Design review of the part shown in the three views and the two pictorial views. Dimensions are in mm from the part's minimum x, y and z. Round coordinates to 2 decimals unless told otherwise and drop trailing zeros. Order: outer loops, then holes, each group sorted by start corner. A loop starts at its lowest first (then second) coordinate and runs counter-clockwise, first axis right, second up.
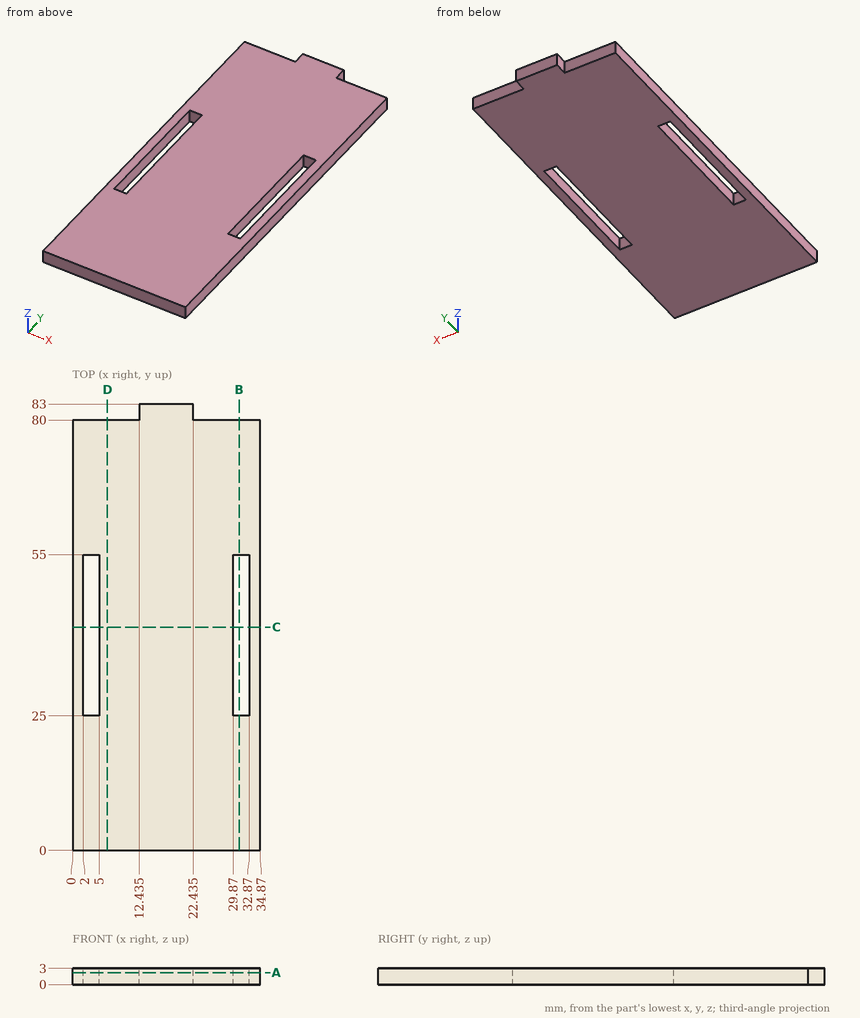
(1) Add section B-B on x = 31. Give the boundary of the cut face in (y, z).
(2) Add section A-A on z = 2.2. Give the boundary of the cut face in (x, y) (3 decimals), plus the area to 3 significant figures.
(3) Clearance check with flat-ended pins moving along their axes: P1, Ø0.9, axis at y = 81, z = 1.5, coming from the +X side (3 decimals); P2, Ø1.5, axis at x = 32, z = 1, coming from the +Y side. State where each tip first meets the part, or that it passes through.
(4) Add section D-D on x = 6.5. Give the boundary of the cut face in (y, z), plus the area to 3 significant figures.
(5) Add section C-C on y = 41.5. Give the boundary of the cut face in (x, z), plus the area to 3 significant figures.
(6) Wall thickness on L1, parallel to X at y = 31.5, z = 2.65; L2, parallel to Y at x = 4.5, z = 2.8; L3, parallel to Y at x = 28, z = 0.8: over which ranges is each line inside the solid? List them lowest first.
Here are the results:
1. outline: (0, 0) - (25, 0) - (25, 3) - (0, 3) - close; (55, 0) - (80, 0) - (80, 3) - (55, 3) - close
2. outline: (0, 0) - (34.87, 0) - (34.87, 80) - (22.435, 80) - (22.435, 83) - (12.435, 83) - (12.435, 80) - (0, 80) - close; hole (2, 25) - (5, 25) - (5, 55) - (2, 55) - close; hole (29.87, 25) - (32.87, 25) - (32.87, 55) - (29.87, 55) - close
2. area: 2,640 mm2
3. P1: stops at x = 22.435
3. P2: stops at y = 80
4. outline: (0, 0) - (80, 0) - (80, 3) - (0, 3) - close
4. area: 240 mm2
5. outline: (0, 0) - (2, 0) - (2, 3) - (0, 3) - close; (5, 0) - (29.87, 0) - (29.87, 3) - (5, 3) - close; (32.87, 0) - (34.87, 0) - (34.87, 3) - (32.87, 3) - close
5. area: 86.6 mm2
6. L1: x = 0 to 2, 5 to 29.87, 32.87 to 34.87
6. L2: y = 0 to 25, 55 to 80
6. L3: y = 0 to 80
